CAD build for the part. Positions are in the model's coordinates, mm. Give positions to 0.01 mm unless a question says otherwise; leave off trailing zeros. Write each loop counter-clockwise with the first axis right and the second up, starting at its lowest first coordinate (ties: lowest second). Pieces come first, ordered by that corner, then holes. Notation, with made-up numbers: M 22.5,50 L 29.5,50 A8 cw 29.5,56 Z; hole C 2.25,16 d8. An arc over 180 degrees is marked long. One line per question, with ' | ' between items. Start each with the question number.
1. Cut at D-D, the plane x = 25.5. Write the cut outline in (y, z), then the cut area to 3 significant figures.
2. Cut at A-A, the plane x = 0. Write the cut outline in (y, z), then the cut area to 3 significant figures.
3. Wall check: L1, parallel to X at y = 1.8, z = 0; L2, parallel to X at y = 2.35, z = -2; L3, parallel to X at y = 2.6, z = -8. Give the ranges that are in metal, low to high.
4. Cut at B-B, the plane z = 0. Write the cut outline in (x, y), then the cut area to 3 significant figures.
5. Flat gauge pins, fed straight in: pin 1 (4 mm diameter, centred on x = -1, z = -16, fed in from +Y); pin 2 (1 mm diameter, centred on x = 25.5, y = 2, fed in from +Z); pin 3 (1 mm diameter, centred on y = 3, z = -25.5, fed in from +X). Where does each tip first touch, or does it go through?
6. Cut at C-C, the plane y = 3. Count the separate pieces of the cut face and the enclosed holes in it, then the cut area to 3 significant figures.
```python
from build123d import *

# Parameters (mm, degrees)
SKETCH1_R             = 42.5
BOSS_EXTRUDE1_DEPTH   = 4
SKETCH2_R             = 5
CUT_EXTRUDE1_DEPTH    = 61.237031799
SKETCH3_R             = 4.028837432
CUT_EXTRUDE2_DEPTH    = 3.872215
CIRPATTERN1_START     = 0.127785179
CIRPATTERN1_OUTLINE_R = 4.028837432
CIRPATTERN1_DEPTH     = 3.872214821


# Read off the part's stored shape, not the designer's step: CirPattern1
with BuildPart() as part:
    # Sketch1 → Boss-Extrude1 (new body)
    with BuildSketch(Plane(origin=(0, 0, 0), x_dir=(1, 0, 0), z_dir=(0, 1, 0))):
        with Locations(Location((0, 0, 0), (0, 0, 270))):
            Circle(SKETCH1_R)
    extrude(amount=BOSS_EXTRUDE1_DEPTH)

    # Sketch2 → Cut-Extrude1 (cut, through all)
    with BuildSketch(Plane(origin=(0, 0, 0), x_dir=(1, 0, 0), z_dir=(0, 1, 0))):
        with Locations(Location((0, 0, 0), (0, 0, 270))):
            Circle(SKETCH2_R)
    extrude(amount=CUT_EXTRUDE1_DEPTH, mode=Mode.SUBTRACT)

    # Sketch3 → Cut-Extrude2 (cut)
    with BuildSketch(Plane(origin=(0, 4, 0), x_dir=(1, 0, 0), z_dir=(0, 1, 0))):
        with Locations(Location((-15.691767503, 0, 0), (0, 0, 270))):
            Circle(SKETCH3_R)
    extrude(amount=-CUT_EXTRUDE2_DEPTH, mode=Mode.SUBTRACT)

    # CirPattern1 outline → CirPattern1 (cut)
    with BuildSketch(Plane(origin=(0, 0, 0), x_dir=(1, 0, 0), z_dir=(0, 1, 0)).offset(CIRPATTERN1_START)):
        with Locations((-11.09575521, -11.09575521)):
            Circle(CIRPATTERN1_OUTLINE_R)
        with Locations((-11.09575521, 11.09575521)):
            Circle(CIRPATTERN1_OUTLINE_R)
        with Locations((0, 15.691767503)):
            Circle(CIRPATTERN1_OUTLINE_R)
        with Locations((11.09575521, 11.09575521)):
            Circle(CIRPATTERN1_OUTLINE_R)
        with Locations((15.691767503, 0)):
            Circle(CIRPATTERN1_OUTLINE_R)
        with Locations((11.09575521, -11.09575521)):
            Circle(CIRPATTERN1_OUTLINE_R)
        with Locations((0, -15.691767503)):
            Circle(CIRPATTERN1_OUTLINE_R)
    extrude(amount=CIRPATTERN1_DEPTH, mode=Mode.SUBTRACT)


solid = part.part
```
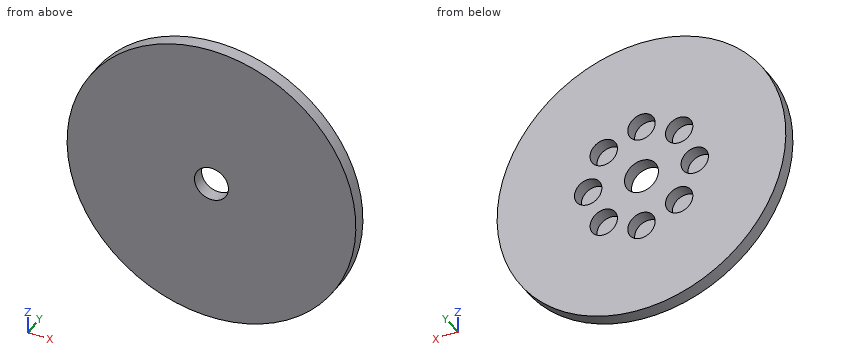
Here are the results:
1) outline: M 0,-34 L 4,-34 L 4,34 L 0,34 Z | area: 272 mm^2
2) outline: M 0,-42.5 L 4,-42.5 L 4,-19.72 L 0.13,-19.72 L 0.13,-11.66 L 4,-11.66 L 4,-5 L 0,-5 Z; M 0,5 L 4,5 L 4,11.66 L 0.13,11.66 L 0.13,19.72 L 4,19.72 L 4,42.5 L 0,42.5 Z | area: 238 mm^2
3) L1: -42.5 to -19.72, -11.66 to -5, 5 to 11.66, 19.72 to 42.5 | L2: -42.45 to -19.19, -12.19 to -4.58, 4.58 to 12.19, 19.19 to 42.45 | L3: -41.74 to -13.67, -8.52 to 8.52, 13.67 to 41.74
4) outline: M -42.5,0 L -5,0 L -5,4 L -11.66,4 L -11.66,0.13 L -19.72,0.13 L -19.72,4 L -42.5,4 Z; M 5,0 L 42.5,0 L 42.5,4 L 19.72,4 L 19.72,0.13 L 11.66,0.13 L 11.66,4 L 5,4 Z | area: 238 mm^2
5) pin 1: y = 0.13 | pin 2: z = 34.37 | pin 3: x = 34.37
6) separate pieces: 1 | enclosed holes: 9 | area: 5,190 mm^2
